Could you check a few things on this model? Use its own coordinates, in mm. Give positions to 0.01 mm unless a question says otherwise; leave off trailing zeros. Loops run counter-clockwise (first coordinate to the right, second up) from the corner with the lowest first, then second, coordinate; pieces in that order, holes last. Notation, with made-up numbers: M 12,-35 L 49,-35 A12 cw 49,-12 Z; hole C -3,59.5 d6. An arc over 180 degrees is marked long. Return JSON: item names as keys, results as strings. Group by question number.
1. For pin 1 (5 mm diameter, centred on y = 34.5, z = 2, fed in from -X); pin 2 (5 mm diameter, centred on y = 29, z = 3, fed in from -X), each with a flat end and sliding along its axis, tell me the tip position at first contact or that it passes through.
2. Please list where these lines run through material, in increasing order: line 1 (Y direction, x = 122.5, z = 9); line 2 (Y direction, x = 180, z = 3.5); line 3 (X direction, y = 74, z = 5.25).
3. If we section it at A-A (y = 75): Write out the boundary of the cut face in (x, z), plus the area to 3 significant figures.
4. If we section it at B-B (x = 255.5): Write out the boundary of the cut face in (y, z), plus the area to 3 significant figures.
Autodesk Inventor part; units mm, degrees
ref_plane "YZ Plane" through (0, 0, 0) normal (1, 0, 0) x (0, 1, 0)
ref_plane "XZ Plane" through (0, 0, 0) normal (0, 1, 0) x (-1, 0, 0)
ref_plane "XY Plane" through (0, 0, 0) normal (0, 0, 1) x (1, 0, 0)
sketch "Sketch1" plane through (0, 0, 0) normal (0, 0, 1) x (1, 0, 0)
  line L0 (75, 0) -> (475, 0)
  line L1 (550, 75) -> (550, 75)
  line L2 (475, 150) -> (75, 150)
  line L3 (0, 75) -> (0, 75)
  arc A0 (75, 150) -> (0, 75) centre (75, 75) ccw
  arc A1 (0, 75) -> (75, 0) centre (75, 75) ccw
  arc A2 (475, 0) -> (550, 75) centre (475, 75) ccw
  arc A3 (550, 75) -> (475, 150) centre (475, 75) ccw
  line L4 (75, 138) -> (475, 138)
  line L5 (538, 75) -> (538, 75)
  line L6 (475, 12) -> (75, 12)
  line L7 (12, 75) -> (12, 75)
  arc A4 (75, 138) -> (12, 75) centre (75, 75) ccw
  arc A5 (12, 75) -> (75, 12) centre (75, 75) ccw
  arc A6 (475, 12) -> (538, 75) centre (475, 75) ccw
  arc A7 (538, 75) -> (475, 138) centre (475, 75) ccw
  point P0 (0, 0)
  point P1 (550, 150)
  point P2 (550, 0)
  point P3 (0, 150)
  point P4 (531, 5)
  point P5 (531, 131)
  point P6 (5, 5)
  point P7 (538, 12)
  point P8 (538, 138)
  point P9 (12, 12)
  dimension "d0" = 550
  dimension "d1" = 150
  dimension "d2" = 75
  dimension "d3" = 526
  dimension "d4" = 126
  dimension "d6" = 526
  dimension "d7" = 126
  dimension "d8" = 63
extrude "Extrusion1" add sketch "Sketch1" along normal blind 16
chamfer "Chamfer1" distance 6 angle 40 4 edges at (275, 12, 16) (30.4523, 30.4523, 16) (275, 138, 16) (519.5477, 119.5477, 16) measured on face at (341.6667, 8, 16)
chamfer "Chamfer2" distance 6 angle 40 4 edges at (275, 138, 0) (30.4523, 30.4523, 0) (275, 12, 0) (519.5477, 119.5477, 0) measured on face at (341.6667, 8, 0)
properties part number "big belt" material "Rubber"
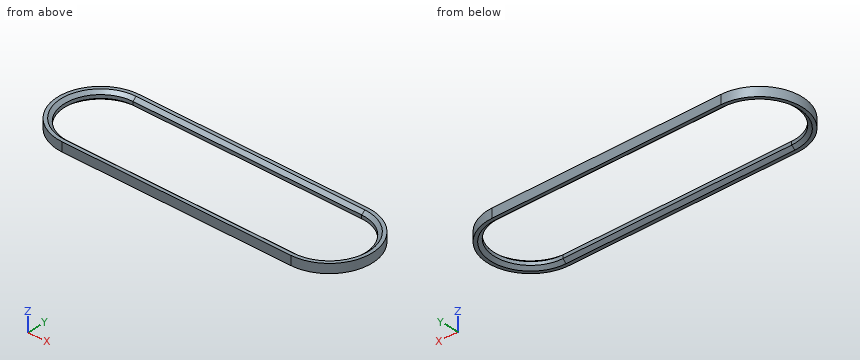
Answer:
{
 "1": {"pin 1": "stops at x = 10.34", "pin 2": "stops at x = 13.9"},
 "2": {"line 1": "y = 0 to 12, 138 to 150", "line 2": "y = 0 to 10.17, 139.83 to 150", "line 3": "x = 0.01 to 12.01, 537.99 to 549.99"},
 "3": {"outline": "M 0,0 L 6,0 L 12,5.03 L 12,10.97 L 6,16 L 0,16 Z; M 538,5.03 L 544,0 L 550,0 L 550,16 L 544,16 L 538,10.97 Z", "area": "324 mm²"},
 "4": {"outline": "M 0,0 L 6,0 L 12,5.03 L 12,10.97 L 6,16 L 0,16 Z; M 138,5.03 L 144,0 L 150,0 L 150,16 L 144,16 L 138,10.97 Z", "area": "324 mm²"}
}
